Model file for the job. Use its own axes, mm. Face numbers are marked on the shaded views. A direction names the side the tool comes from. Round coordinates to 2 decimals unless told otherwise and drop trailing zeros. Loops run counter-clockwise (first coordinate to the right, second up) from the corner with the lowest first, then second, coordinate; pieces in that order, holes last. Notation, with made-up numbers: M -29,76.25 L 17,76.25 A31 ccw 17,114.25 Z; hole C 9.25,-10 d6. An arc over 180 degrees is marked long. Answer in a Markdown table with one row per item.
from build123d import *

# Parameters (mm, degrees)
SKETCH1_W           = 35
SKETCH1_H           = 35
SKETCH1_R           = 5.5
BOSS_EXTRUDE1_DEPTH = 115
CUT_EXTRUDE2_DEPTH  = 30
SKETCH3_W           = 50
SKETCH3_H           = 50
SKETCH3_R           = 5.5
BOSS_EXTRUDE2_DEPTH = 10
SKETCH4_R           = 2.5
CUT_EXTRUDE3_DEPTH  = 15
SKETCH6_R           = 1.05
CUT_EXTRUDE4_DEPTH  = 5
SKETCH7_R           = 1.05
CUT_EXTRUDE5_DEPTH  = 5
SKETCH8_R           = 1.05
CUT_EXTRUDE6_DEPTH  = 5
SKETCH9_R           = 1.05
CUT_EXTRUDE7_DEPTH  = 5
SKETCH11_R          = 1.05
CUT_EXTRUDE8_DEPTH  = 5
SKETCH12_W          = 43
SKETCH12_H          = 23
CUT_EXTRUDE9_DEPTH  = 8
SKETCH13_W          = 40
SKETCH13_H          = 23
CUT_EXTRUDE10_DEPTH = 8
FILLET1_R           = 10
SKETCH14_R          = 5
CUT_EXTRUDE11_DEPTH = 10
CUT_EXTRUDE12_REACH = 44.5
SKETCH15_R          = 2.5


with BuildPart() as part:
    # Sketch1 → Boss-Extrude1 (new body)
    with BuildSketch(Plane(origin=(0, 0, 0), x_dir=(0, 0, -1), z_dir=(1, 0, 0))):
        with Locations((17.5, 17.5)):
            Rectangle(SKETCH1_W, SKETCH1_H)
        with Locations((17.5, 17.5)):
            Circle(SKETCH1_R, mode=Mode.SUBTRACT)
    extrude(amount=BOSS_EXTRUDE1_DEPTH)

    # Sketch2 → Cut-Extrude2 (cut)
    with BuildSketch(Plane(origin=(115, 0, 0), x_dir=(0, 0, -1), z_dir=(1, 0, 0))):
        Polygon((0, 13.553396292), (6, 10.089294677), (6, 25.017497907), (0, 21.553396292), (-1, 21.553396292), (-1, 13.553396292), align=None)
        Polygon((21.5, 35.053396292), (21.5, 36.053396292), (13.5, 36.053396292), (13.5, 35.053396292), (10.035898385, 29.053396292), (24.964101615, 29.053396292), align=None)
        Polygon((35, 13.553396292), (36, 13.553396292), (36, 21.553396292), (35, 21.553396292), (29, 25.017497907), (29, 10.089294677), align=None)
    extrude(amount=-CUT_EXTRUDE2_DEPTH, mode=Mode.SUBTRACT)

    # Sketch3 → Boss-Extrude2 (add)
    with BuildSketch(Plane.ZY):
        with Locations((-17.5, 17.5)):
            Rectangle(SKETCH3_W, SKETCH3_H)
        with Locations((-17.5, 17.5)):
            Circle(SKETCH3_R, mode=Mode.SUBTRACT)
    extrude(amount=BOSS_EXTRUDE2_DEPTH)

    # Sketch4 → Cut-Extrude3 (cut)
    with BuildSketch(Plane.ZY.offset(10)):
        with Locations((-35, 35)):
            Circle(SKETCH4_R)
        with Locations((-35, 0)):
            Circle(SKETCH4_R)
        Circle(SKETCH4_R)
        with Locations((0, 35)):
            Circle(SKETCH4_R)
    extrude(amount=-CUT_EXTRUDE3_DEPTH, mode=Mode.SUBTRACT)

    # Sketch6 → Cut-Extrude4 (cut)
    with BuildSketch(Plane(origin=(0, 0, 0), x_dir=(-1, 0, 0), z_dir=(0, 0, 1))):
        with Locations((-65, -8)):
            Circle(SKETCH6_R)
        with Locations((-73, -8)):
            Circle(SKETCH6_R)
        with Locations((-81, -8)):
            Circle(SKETCH6_R)
        with Locations((-73, -16)):
            Circle(SKETCH6_R)
        with Locations((-81, -16)):
            Circle(SKETCH6_R)
        with Locations((-73, -24)):
            Circle(SKETCH6_R)
        with Locations((-81, -24)):
            Circle(SKETCH6_R)
        with Locations((-65, -16)):
            Circle(SKETCH6_R)
        with Locations((-65, -24)):
            Circle(SKETCH6_R)
    extrude(amount=-CUT_EXTRUDE4_DEPTH, mode=Mode.SUBTRACT)

    # Sketch7 → Cut-Extrude5 (cut)
    with BuildSketch(Plane(origin=(0, 35, 0), x_dir=(-1, 0, 0), z_dir=(0, 1, 0))):
        with Locations((-65, -8)):
            Circle(SKETCH7_R)
        with Locations((-73, -8)):
            Circle(SKETCH7_R)
        with Locations((-81, -8)):
            Circle(SKETCH7_R)
        with Locations((-73, -16)):
            Circle(SKETCH7_R)
        with Locations((-81, -16)):
            Circle(SKETCH7_R)
        with Locations((-73, -24)):
            Circle(SKETCH7_R)
        with Locations((-81, -24)):
            Circle(SKETCH7_R)
        with Locations((-65, -16)):
            Circle(SKETCH7_R)
        with Locations((-65, -24)):
            Circle(SKETCH7_R)
    extrude(amount=-CUT_EXTRUDE5_DEPTH, mode=Mode.SUBTRACT)

    # Sketch8 → Cut-Extrude6 (cut)
    with BuildSketch(Plane(origin=(0, 0, -35), x_dir=(1, 0, 0), z_dir=(0, 0, -1))):
        with Locations((81, -11)):
            Circle(SKETCH8_R)
        with Locations((73, -11)):
            Circle(SKETCH8_R)
        with Locations((65, -11)):
            Circle(SKETCH8_R)
        with Locations((73, -19)):
            Circle(SKETCH8_R)
        with Locations((65, -19)):
            Circle(SKETCH8_R)
        with Locations((73, -27)):
            Circle(SKETCH8_R)
        with Locations((65, -27)):
            Circle(SKETCH8_R)
        with Locations((81, -19)):
            Circle(SKETCH8_R)
        with Locations((81, -27)):
            Circle(SKETCH8_R)
    extrude(amount=-CUT_EXTRUDE6_DEPTH, mode=Mode.SUBTRACT)

    # Sketch9 → Cut-Extrude7 (cut)
    with BuildSketch(Plane.XZ):
        with Locations((56, -11)):
            Circle(SKETCH9_R)
        with Locations((48, -11)):
            Circle(SKETCH9_R)
        with Locations((40, -11)):
            Circle(SKETCH9_R)
        with Locations((48, -19)):
            Circle(SKETCH9_R)
        with Locations((40, -19)):
            Circle(SKETCH9_R)
        with Locations((48, -27)):
            Circle(SKETCH9_R)
        with Locations((40, -27)):
            Circle(SKETCH9_R)
        with Locations((56, -19)):
            Circle(SKETCH9_R)
        with Locations((56, -27)):
            Circle(SKETCH9_R)
    extrude(amount=-CUT_EXTRUDE7_DEPTH, mode=Mode.SUBTRACT)

    # Sketch11 → Cut-Extrude8 (cut)
    with BuildSketch(Plane(origin=(0, 35, 0), x_dir=(-1, 0, 0), z_dir=(0, 1, 0))):
        with Locations((-10, -11)):
            Circle(SKETCH11_R)
        with Locations((-18, -11)):
            Circle(SKETCH11_R)
        with Locations((-26, -11)):
            Circle(SKETCH11_R)
        with Locations((-18, -19)):
            Circle(SKETCH11_R)
        with Locations((-26, -19)):
            Circle(SKETCH11_R)
        with Locations((-18, -27)):
            Circle(SKETCH11_R)
        with Locations((-26, -27)):
            Circle(SKETCH11_R)
        with Locations((-10, -19)):
            Circle(SKETCH11_R)
        with Locations((-10, -27)):
            Circle(SKETCH11_R)
    extrude(amount=-CUT_EXTRUDE8_DEPTH, mode=Mode.SUBTRACT)

    # Sketch12 → Cut-Extrude9 (cut)
    with BuildSketch(Plane.XY):
        with Locations((33.5, 17.5)):
            Rectangle(SKETCH12_W, SKETCH12_H)
    extrude(amount=-CUT_EXTRUDE9_DEPTH, mode=Mode.SUBTRACT)

    # Sketch13 → Cut-Extrude10 (cut)
    with BuildSketch(Plane(origin=(0, 0, -35), x_dir=(-1, 0, 0), z_dir=(0, 0, -1))):
        with Locations((-35, 17.5)):
            Rectangle(SKETCH13_W, SKETCH13_H)
    extrude(amount=-CUT_EXTRUDE10_DEPTH, mode=Mode.SUBTRACT)

    # Fillet1
    fillet1_edges = [part.edges().sort_by_distance(p)[0] for p in [
        (-5, -7.5, 7.5),
        (-5, 42.5, 7.5),
        (-5, 42.5, -42.5),
        (-5, -7.5, -42.5),
    ]]
    fillet(fillet1_edges, radius=FILLET1_R)

    # Sketch14 → Cut-Extrude11 (cut)
    with BuildSketch(Plane(origin=(0, 0, 0), x_dir=(0, 0, -1), z_dir=(1, 0, 0))):
        Circle(SKETCH14_R)
        with Locations((35, 0)):
            Circle(SKETCH14_R)
        with Locations((35, 35)):
            Circle(SKETCH14_R)
        with Locations((0, 35)):
            Circle(SKETCH14_R)
    extrude(amount=CUT_EXTRUDE11_DEPTH, mode=Mode.SUBTRACT)

    # Sketch15 → Cut-Extrude12 (cut, up to next)
    with BuildSketch(Plane.XZ, mode=Mode.PRIVATE) as cut_extrude12_sk1:
        with Locations((100, -17.5)):
            Circle(SKETCH15_R)
    cut_extrude12_tool1 = extrude(cut_extrude12_sk1.sketch, amount=-CUT_EXTRUDE12_REACH, mode=Mode.PRIVATE) & part.part
    add(cut_extrude12_tool1.solids().sort_by_distance((100, 0, -17.5))[0], mode=Mode.SUBTRACT)


solid = part.part
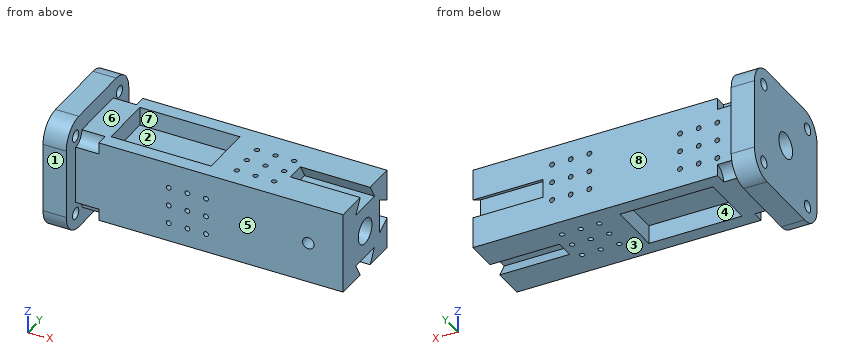
1. Saw through at A-A (x = 53.5). Write the cut outline in (y, z), and give its area (3 significant figures).
Verdict:
| item | result |
|---|---|
| outline | M 0,-35 L 6,-35 L 6,-27 L 29,-27 L 29,-35 L 35,-35 L 35,0 L 29,0 L 29,-8 L 6,-8 L 6,0 L 0,0 Z; hole C 17.5,-17.5 d11 |
| area | 762 mm² |
2. Tool access for the marked faces 5, 6, 7 and 8: list every direction of +Z, -Z, +X, -X, +Y, -Y with a clear straight run to the whole face (end or side of a thin tool).
Verdict:
| item | result |
|---|---|
| face 5 | +Z, -Z, +X, -Y |
| face 6 | +Z, +X, +Y, -Y |
| face 7 | +Z |
| face 8 | +Z, -Z, +X, +Y |
3. Saw through at B-B (x = 70.5). Write the cut outline in (y, z).
Verdict:
| item | result |
|---|---|
| outline | M 0,-35 L 35,-35 L 35,0 L 0,0 Z; hole C 17.5,-17.5 d11 |
4. Mould opens along Y. For the marked faces 1, 2, 3 and 4 say: +Y half, -Y half, draft (parallel to the pull), parting line (faces both ways), or undercut.
Verdict:
| item | result |
|---|---|
| face 1 | -Y half |
| face 2 | undercut |
| face 3 | draft |
| face 4 | undercut |
5. Wall check: probe 1 along X at (y, z) = (8, -1.15); probe 2 along X at (y, z) = (16, -1.65); probe 3 along Z at (x, y) = (51.5, 17.5). Give the ranges that are in metal, low to high.
Verdict:
| item | result |
|---|---|
| probe 1 | x = -10 to 12, 55 to 63.95, 66.05 to 71.95, 74.05 to 79.95, 82.05 to 115 |
| probe 2 | x = -10 to 12, 55 to 63.95, 66.05 to 71.95, 74.05 to 79.95, 82.05 to 85 |
| probe 3 | z = -27 to -23, -12 to -8 |
6. Pin check, flat tips, straight feed: pin 1 (1.3 mm diameter, centred on x = 18, z = -19, fed in from +Y); pin 2 (2.5 mm diameter, centred on x = 81, y = 24, fed in from -Z); pin 3 (2.5 mm diameter, centred on x = 42.5, z = -2.5, fed in from +Y). Stop position of each tip, or through.
Verdict:
| item | result |
|---|---|
| pin 1 | stops at y = 30 |
| pin 2 | stops at z = -35 |
| pin 3 | stops at y = 35 |
